Part model, mm, in its own coordinate system. A direction names the side the tool comes from. Give positions to 0.01 mm unless a question says otherwise; leave off trailing zeros. Write each loop counter-clockwise with the first axis right and the second up, starting at its lowest first coordinate (ties: lowest second). Pieces come first, ordered by that corner, then holes.
```python
from build123d import *

# Parameters (mm, degrees)
SKETCH1_W           = 100
SKETCH1_H           = 50
BOSS_EXTRUDE1_DEPTH = 50
FILLET1_R           = 10
SHELL1_T            = -5
SKETCH2_R           = 2.5
CUT_EXTRUDE1_DEPTH  = 115.564392374


with BuildPart() as part:
    # Sketch1 → Boss-Extrude1 (new body)
    with BuildSketch(Plane(origin=(0, 0, 0), x_dir=(1, 0, 0), z_dir=(0, 1, 0))):
        Rectangle(SKETCH1_W, SKETCH1_H)
    extrude(amount=BOSS_EXTRUDE1_DEPTH)

    # Fillet1
    fillet1_edges = [part.edges().sort_by_distance(p)[0] for p in [
        (-50, 25, -25),
        (50, 25, -25),
        (50, 25, 25),
        (-50, 25, 25),
    ]]
    fillet(fillet1_edges, radius=FILLET1_R)

    # Shell1
    shell1_openings = [part.faces().sort_by_distance(p)[0] for p in [
        (0, 50, 0),
    ]]
    offset(amount=SHELL1_T, openings=shell1_openings, kind=Kind.INTERSECTION)

    # Sketch2 → Cut-Extrude1 (cut, through all)
    with BuildSketch(Plane(origin=(50, 0, 0), x_dir=(0, 0, -1), z_dir=(1, 0, 0))):
        with Locations((0, 40)):
            Circle(SKETCH2_R)
    extrude(amount=-CUT_EXTRUDE1_DEPTH, mode=Mode.SUBTRACT)


solid = part.part
```
1) Wall check: L1, parallel to Y at x = 47.1, z = 0; L2, parallel to Z at x = 37, y = 35; L3, parallel to X at y = 39, z = -5. Give the ranges that are in metal, low to high.
Answers follow:
L1: y = 0 to 37.5, 42.5 to 50
L2: z = -25 to -20, 20 to 25
L3: x = -50 to -45, 45 to 50
2) Saw through at C-C, the plane x = 22. Write the cut outline in (y, z).
Answers follow:
outline: (0, -25) - (50, -25) - (50, -20) - (5, -20) - (5, 20) - (50, 20) - (50, 25) - (0, 25) - close
3) Two-plate mould, pull along Z, no slides. Class faces 3 (the face through (-1, 0, 0)), 4 (the face through (-1, 25, -25)), 5 (the face through (-1, 25, 25)), 6 (the face through (45, 27, 0)): +Z half, -Z half, draft (parallel to the pull), parting line (faces both ways), or undercut.
Answers follow:
face 3: draft
face 4: -Z half
face 5: +Z half
face 6: undercut
4) 3-axis set-ups, long thin cutter, end or side, ignore diameter. For faces 1 (the face through (50, 25, 0)), 2 (the face through (-1, 27, -20)): which of +Z, -Z, +X, -X, +Y, -Y reach the whole face in a straight line?
Answers follow:
face 1: +Z, -Z, +X, +Y, -Y
face 2: +Y
5) Saw through at D-D, the plane y = 46. Write the cut outline in (x, z), then the cut area to 3 significant figures.
Answers follow:
outline: (-50, -15) arc R10 ccw to (-40, -25) - (40, -25) arc R10 ccw to (50, -15) - (50, 15) arc R10 ccw to (40, 25) - (-40, 25) arc R10 ccw to (-50, 15) - close; hole (-45, -15) arc R5 ccw to (-40, -20) - (40, -20) arc R5 ccw to (45, -15) - (45, 15) arc R5 ccw to (40, 20) - (-40, 20) arc R5 ccw to (-45, 15) - close
area: 1,340 mm2
6) Pin check, flat tips, straight feed: pin 1 Ø4.5 at (y, z) = (40, 0) entering from -X; pin 2 Ø8 at (x, z) = (35.5, -3) entering from +Y. Stop position of each tip, or through.
Answers follow:
pin 1: passes through
pin 2: stops at y = 5
7) Saw through at A-A, the plane z = 0. Write the cut outline in (x, y).
Answers follow:
outline: (-50, 0) - (50, 0) - (50, 37.5) - (45, 37.5) - (45, 5) - (-45, 5) - (-45, 37.5) - (-50, 37.5) - close; (-50, 42.5) - (-45, 42.5) - (-45, 50) - (-50, 50) - close; (45, 42.5) - (50, 42.5) - (50, 50) - (45, 50) - close
8) Saw through at B-B, the plane y = 40. Write the cut outline in (x, z), then the cut area to 3 significant figures.
Answers follow:
outline: (-50, -15) arc R10 ccw to (-40, -25) - (40, -25) arc R10 ccw to (50, -15) - (50, -2.5) - (45, -2.5) - (45, -15) arc R5 cw to (40, -20) - (-40, -20) arc R5 cw to (-45, -15) - (-45, -2.5) - (-50, -2.5) - close; (-50, 2.5) - (-45, 2.5) - (-45, 15) arc R5 cw to (-40, 20) - (40, 20) arc R5 cw to (45, 15) - (45, 2.5) - (50, 2.5) - (50, 15) arc R10 ccw to (40, 25) - (-40, 25) arc R10 ccw to (-50, 15) - close
area: 1,290 mm2
